Design review of the part built by this model. Coordinates are the model's own, in mm. A direction names the side the tool comes from. Coordinates: 2 decimals unless noted, no trailing zeros. Order: outer loops, then holes, each group sorted by start corner. A loop starts at its lowest first (then second) coordinate and runs counter-clockwise, first axis right, second up. Notation, with made-up numbers: M -5,-7.5 L -1,-7.5 A21 cw -1,12.5 Z; hole C 59.5,-15 d4. An arc over 180 degrees is marked long. Answer in a Markdown table with one row per item.
from build123d import *

# Parameters (mm, degrees)
SKETCH7_R            = 35
BOSS_EXTRUDE6_DEPTH  = 20
SKETCH6_R            = 16.1
DISPLAY_CUTOUT_DEPTH = 54.38539126
SKETCH1_R            = 16.1
CUT_EXTRUDE6_DEPTH   = 7
FILLET2_R            = 4
FILLET3_R            = 1
SKETCH8_R            = 27
CUT_EXTRUDE7_DEPTH   = 9
CHAMFER1_SIZE        = 1
FILLET4_R            = 0.5
SKETCH9_R            = 19.85
SKETCH9_R_2          = 17.85
EXTRUDE_THIN1_DEPTH  = 1
FILLET5_R            = 1


with BuildPart() as part:
    # Sketch7 → Boss-Extrude6 (new body)
    with BuildSketch(Plane(origin=(0, 0, 0), x_dir=(1, 0, 0), z_dir=(0, 1, 0))):
        with Locations(Location((0, 0, 0), (0, 0, 270))):
            Circle(SKETCH7_R)
    extrude(amount=BOSS_EXTRUDE6_DEPTH)

    # Sketch6 → Display cutout (cut, through all)
    with BuildSketch(Plane(origin=(0, 0, 0), x_dir=(1, 0, 0), z_dir=(0, 1, 0))):
        with Locations(Location((0, 0, 0), (0, 0, 270))):
            Circle(SKETCH6_R)
    extrude(amount=DISPLAY_CUTOUT_DEPTH, mode=Mode.SUBTRACT)

    # Sketch1 → Cut-Extrude6 (cut)
    with BuildSketch(Plane(origin=(0, 0, 0), x_dir=(1, 0, 0), z_dir=(0, 1, 0))):
        with BuildLine():
            Line((2.04, -30), (2.04, -28.928159292))
            ThreePointArc((2.04, -28.928159292), (25.11473671, -14.5), (26.072520831, 12.697387822))
            Line((26.072520831, 12.697387822), (27.000762114, 13.233308176))
            Line((27.000762114, 13.233308176), (24.960762114, 16.766691824))
            Line((24.960762114, 16.766691824), (24.032520831, 16.23077147))
            ThreePointArc((24.032520831, 16.23077147), (0, 29), (-24.032520831, 16.23077147))
            Line((-24.032520831, 16.23077147), (-24.960762114, 16.766691824))
            Line((-24.960762114, 16.766691824), (-27.000762114, 13.233308176))
            Line((-27.000762114, 13.233308176), (-26.072520831, 12.697387822))
            ThreePointArc((-26.072520831, 12.697387822), (-25.11473671, -14.5), (-2.04, -28.928159292))
            Line((-2.04, -28.928159292), (-2.04, -30))
            Line((-2.04, -30), (2.04, -30))
        make_face()
        with Locations(Location((0, 0, 0), (0, 0, 270))):
            Circle(SKETCH1_R, mode=Mode.SUBTRACT)
    extrude(amount=CUT_EXTRUDE6_DEPTH, mode=Mode.SUBTRACT)

    # Fillet2
    fillet2_edges = [part.edges().sort_by_distance(p)[0] for p in [
        (0, 20, -35),
    ]]
    fillet(fillet2_edges, radius=FILLET2_R)

    # Fillet3
    fillet3_edges = [part.edges().sort_by_distance(p)[0] for p in [
        (0, 20, -16.1),
    ]]
    fillet(fillet3_edges, radius=FILLET3_R)

    # Sketch8 → Cut-Extrude7 (cut)
    with BuildSketch(Plane.XZ.offset(-7)):
        with Locations(Location((0, 0, 0), (0, 0, 270))):
            Circle(SKETCH8_R)
    extrude(amount=-CUT_EXTRUDE7_DEPTH, mode=Mode.SUBTRACT)

    # Chamfer1
    chamfer1_edges = [part.edges().sort_by_distance(p)[0] for p in [
        (0, 0, -35),
    ]]
    chamfer(chamfer1_edges, length=CHAMFER1_SIZE)

    # Fillet4
    fillet4_edges = [part.edges().sort_by_distance(p)[0] for p in [
        (2.04, 3.5, 28.928159292),
        (24.032520831, 3.5, -16.23077147),
        (-26.072520831, 3.5, -12.697387822),
        (-2.04, 3.5, 28.928159292),
        (-24.032520831, 3.5, -16.23077147),
        (26.072520831, 3.5, -12.697387822),
    ]]
    fillet(fillet4_edges, radius=FILLET4_R)

    # Sketch9 → Extrude-Thin1 (add)
    with BuildSketch(Plane.XZ.offset(-16)):
        Circle(SKETCH9_R)
        Circle(SKETCH9_R_2, mode=Mode.SUBTRACT)
    extrude(amount=EXTRUDE_THIN1_DEPTH)

    # Fillet5
    fillet5_edges = [part.edges().sort_by_distance(p)[0] for p in [
        (-17.85, 15, 0),
    ]]
    fillet(fillet5_edges, radius=FILLET5_R - 0.0001)  # a hair under: the kernel refuses the full size


solid = part.part
(1) Draft analysis for pull direction Z (two halves, no side actions). For faces 1 (the flat face through (15, 0, 25)), 2 (the cylindrical face through (-21, 8, -28)), 3 (the cylindrical face through (-26.36, 11.44, 5.85)), state which applies: pulls with the +Z half, pulls with the -Z half, needs draft (parallel to the pull), parting line crosses it, or undercut.
Return value:
| item | result |
|---|---|
| face 1 | needs draft |
| face 2 | parting line crosses it |
| face 3 | undercut |
(2) Add section C-C, the plane y = 5.25. Give the boundary of the cut face in (x, z).
Return value:
| item | result |
|---|---|
| outline | C 0,0 d70; hole M -27,-13.23 L -24.96,-16.77 L -24.43,-16.46 A0.5 cw -23.77,-16.61 A29 ccw 23.77,-16.61 A0.5 cw 24.43,-16.46 L 24.96,-16.77 L 27,-13.23 L 26.47,-12.93 A0.5 cw 26.27,-12.28 A29 ccw 2.5,28.89 A0.5 cw 2.04,29.39 L 2.04,30 L -2.04,30 L -2.04,29.39 A0.5 cw -2.5,28.89 A29 ccw -26.27,-12.28 A0.5 cw -26.47,-12.93 Z |
(3) Insertion check: pin 1 Ø12 at (x, y) = (-12.5, 13) entering from +Z; pin 2 Ø1 at (x, y) = (25.5, 7) entering from -Z; pin 3 Ø16 at (x, z) = (-5, -11) entering from -Y. Each pin has a flat end and moves straight along its axis. Give the tip position at first contact, or say it passes through.
Return value:
| item | result |
|---|---|
| pin 1 | stops at z = 34.39 |
| pin 2 | stops at z = -24.49 |
| pin 3 | stops at y = 15 |
(4) For line 1 along X through (y, z) = (12.75, 0); line 2 along Y through (x, z) = (28, -6); line 3 along X through (y, z) = (18, 14), list the stretches that pass through material, from the lowest coordinate up. Write a range as from..to.
Return value:
| item | result |
|---|---|
| line 1 | x = -35..-27, 27..35 |
| line 2 | y = 7..20 |
| line 3 | x = -31.49..-7.95, 7.95..31.49 |
(5) For faces 4 (the flat face through (20.1, 16, 0.1)), 5 (the cylindrical face through (-6.17, 17.48, 14.87)), list the 3-axis set-ups (+Z, -Z, +X, -X, +Y, -Y) from which the entire face can be reached by the end or side of a thin tool; tool diameter is ignored.
Return value:
| item | result |
|---|---|
| face 4 | -Y |
| face 5 | +Y, -Y |
